Design review of the part built by this model. Coordinates are the model's own, in mm. A direction names the side the tool comes from. Coordinates: 2 decimals unless noted, no trailing zeros. Loops run counter-clockwise (first coordinate to the right, second up) from the corner with the lowest first, then second, coordinate; pieces in that order, holes last. Notation, with made-up numbers: (43, -5.5) -> (78, -5.5) arc R10 ccw to (78, 6.5) -> close; hole circle Ø6 at (31, 73.5). An arc over 180 degrees is marked (long way). Use CSV: the item, a comma, the result in double quotes.
```python
from build123d import *

# Parameters (mm, degrees)
F0_W     = 50.8
F0_H     = 50.8
F1_DEPTH = 876.3
F2_W     = 44.45
F2_H     = 44.45
F3_DEPTH = 876.3
F4_R     = 9.525
F5_R     = 12.7
F6_DEPTH = 50.8


with BuildPart() as f1:
    # F0 (on Right) → F1 (new body)
    with BuildSketch(Plane.YZ):
        with Locations((25.4, 25.4)):
            Rectangle(F0_W, F0_H)
    extrude(amount=-F1_DEPTH)

    # F2 (on face) → F3 (cut)
    with BuildSketch(Plane.YZ):
        with Locations((25.4, 25.4)):
            Rectangle(F2_W, F2_H)
    extrude(amount=-F3_DEPTH, mode=Mode.SUBTRACT)

    # F4
    f4_edges = [f1.edges().sort_by_distance(p)[0] for p in [
        (-438.15, 3.175, 3.175),
        (-438.15, 47.625, 3.175),
        (-438.15, 47.625, 47.625),
        (-438.15, 3.175, 47.625),
        (-438.15, 50.8, 0),
        (-438.15, 50.8, 50.8),
        (-438.15, 0, 50.8),
        (-438.15, 0, 0),
    ]]
    fillet(f4_edges, radius=F4_R)

    # F5 (on face) → F6 (cut)
    with BuildSketch(Plane.XY.offset(50.8)):
        with Locations((-844.55, 25.4)):
            Circle(F5_R)
    extrude(amount=-F6_DEPTH, mode=Mode.SUBTRACT)


solid = f1.part
```
Item 1: Machinability: for faces 1 (the face through (0, 27, 3)), 2 (the face through (-432, 47.625, 25)), which of the approach directions +Z, -Z, +X, -X, +Y, -Y give a long, thin tool a straight path to every point of the face, cutting with its end or side? Answer none if there is none.
Checked values:
face 1,"+Z, -Z, +X, +Y, -Y"
face 2,"+X, -X"
Item 2: To check wall thickness, follow line 1 along Z through (x, y) = (-56, 16) (3 decimals); line 2 along X through (y, z) = (25.4, 0.85); line 3 along Y through (x, z) = (-844.55, 2.35). State the ranges of each line that lie inside material, in increasing order.
Checked values:
line 1,"0 to 3.175, 47.625 to 50.8"
line 2,"-876.3 to -857.25, -831.85 to 0"
line 3,"3.26 to 12.7, 38.1 to 47.54"
Item 3: Add section A-A (x = -736.5). Give the boundary of the cut face in (y, z) (3 decimals).
Checked values:
outline,"(0, 9.525) arc R9.525 ccw to (9.525, 0) -> (41.275, 0) arc R9.525 ccw to (50.8, 9.525) -> (50.8, 41.275) arc R9.525 ccw to (41.275, 50.8) -> (9.525, 50.8) arc R9.525 ccw to (0, 41.275) -> close; hole (3.175, 12.7) arc R9.525 ccw to (12.7, 3.175) -> (38.1, 3.175) arc R9.525 ccw to (47.625, 12.7) -> (47.625, 38.1) arc R9.525 ccw to (38.1, 47.625) -> (12.7, 47.625) arc R9.525 ccw to (3.175, 38.1) -> close"
Item 4: Draft analysis for pull direction X (two halves, no side actions). For faces 3 (the face through (-416, 25, 47.625)), 4 (the face through (-853.91, 33.983, 49.235)), 5 (the face through (-876.3, 27, 3)), state which applies: pulls with the +X half, pulls with the -X half, needs draft (parallel to the pull), parting line crosses it, or undercut.
Checked values:
face 3,"needs draft"
face 4,"undercut"
face 5,"pulls with the -X half"
Item 5: Clearance check with flat-ended pins moving along their axes: pin 1 (1.5 mm diameter, centred on x = -315, z = 42.5, fed in from +Y); pin 2 (1.5 mm diameter, centred on x = -104, z = 7.5, fed in from -Y); pin 3 (1 mm diameter, centred on x = -499, z = 7, fed in from +Y). State where each tip first meets the part, or that it passes through.
Checked values:
pin 1,"y = 50.79"
pin 2,"y = 0.09"
pin 3,"y = 50.58"
Item 6: Add section B-B (y = 25.4). Give the boundary of the cut face in (x, z) (3 decimals).
Checked values:
outline,"(-876.3, 0) -> (-857.25, 0) -> (-857.25, 3.175) -> (-876.3, 3.175) -> close; (-876.3, 47.625) -> (-857.25, 47.625) -> (-857.25, 50.8) -> (-876.3, 50.8) -> close; (-831.85, 0) -> (0, 0) -> (0, 3.175) -> (-831.85, 3.175) -> close; (-831.85, 47.625) -> (0, 47.625) -> (0, 50.8) -> (-831.85, 50.8) -> close"
